```python
from build123d import *


with BuildPart() as f1:
    # F0 (on Right) → F1 (revolve)
    with BuildSketch(Plane.YZ):
        with BuildLine():
            Line((-6.35, -10.473485), (-5.488451, -10.473485))
            Line((-5.488451, -10.473485), (-5.488451, -3.844697))
            Line((-5.488451, -3.844697), (0, -3.844697))
            Line((0, -3.844697), (0, -1.438863))
            Line((0, -1.438863), (-10.85, -1.438863))
            ThreePointArc((-10.85, -1.438863), (-11.91066, -1.878203), (-12.35, -2.938863))
            Line((-12.35, -2.938863), (-12.35, -3.438863))
            Line((-12.35, -3.438863), (-6.35, -3.438863))
            Line((-6.35, -3.438863), (-6.35, -6.318287))
            Line((-6.35, -6.318287), (-6.35, -9.81605))
            Line((-6.35, -9.81605), (-6.35, -10.473485))
        make_face()
        Polygon((-6.45, -7.265888), (-6.35, -9.81605), (-6.35, -6.318287), align=None)
    revolve(axis=Axis((0, 0, 16.107956), (0, 0, 1)))


solid = f1.part
```
Model file for the job. Use its own axes, mm. A direction names the side the tool comes from. Give positions to 0.01 mm unless a question says otherwise; leave off trailing zeros. Loops run counter-clockwise (first coordinate to the right, second up) from the corner with the lowest first, then second, coordinate; pieces in that order, holes last. Notation, with made-up numbers: (-2, 15) -> (17, 15) arc R24 cw to (17, 46) -> close; hole circle Ø4 at (64, 86.25). An arc over 180 degrees is marked (long way). Use CSV: the item, a comma, the result in double quotes. Start each with the question number.
1) Slice it at C-C on z = -7.75. Give the cut face in (x, y).
2) Slice it at A-A on y = 0. Give the cut face in (x, z), plus the area to 3 significant figures.
3) Tool access for faces 1 (the cylindrical face through (3.71, -11.78, -3.19)), 2 (the cylindrical face through (-6.2, 1.38, -10.15)), 3 (the cylindrical face through (-6.2, 1.38, -4.9)): list every direction of +Z, -Z, +X, -X, +Y, -Y with a clear straight run to the whole face (end or side of a thin tool).
4) Mould opens along Y. For faces 4 (the flat face through (3, 6, -3.439)), 5 (the cylindrical face through (1.649, -5.235, -7.113)), 6 (the conical face through (-3.887, 5.069, -8.842)) say: released by +Y, released by -Y, zero draft, split by the parting line, or undercut.
5) Wall check: line 1 (Y direction, x = -1.5, z = -7.25); line 2 (Z direction, x = 2.25, y = 0.25); line 3 (X direction, y = 4.75, z = -7). Give the ranges that are in metal, low to high.
6) Flat gauge pins, fed straight in: pin 1 Ø3 at (y, z) = (-4, -2.5) entering from -X; pin 2 Ø3.5 at (x, y) = (1.5, 2.5) entering from -Z. Where does each tip first touch, or does it go through?
Computed values:
1,outline,"circle Ø12.86 at (0, 0); hole circle Ø10.98 at (0, 0)"
2,outline,"(-12.35, -3.44) -> (-6.35, -3.44) -> (-6.35, -6.32) -> (-6.45, -7.27) -> (-6.35, -9.82) -> (-6.35, -10.47) -> (-5.49, -10.47) -> (-5.49, -3.84) -> (5.49, -3.84) -> (5.49, -10.47) -> (6.35, -10.47) -> (6.35, -9.82) -> (6.45, -7.27) -> (6.35, -6.32) -> (6.35, -3.44) -> (12.35, -3.44) -> (12.35, -2.94) arc R1.5 ccw to (10.85, -1.44) -> (-10.85, -1.44) arc R1.5 ccw to (-12.35, -2.94) -> close"
2,area,"65.4 mm^2"
3,face 1,"+Z, -Z"
3,face 2,"-Z"
3,face 3,"none"
4,face 4,"zero draft"
4,face 5,"undercut"
4,face 6,"split by the parting line"
5,line 1,"y = -6.27 to -5.28, 5.28 to 6.27"
5,line 2,"z = -3.84 to -1.44"
5,line 3,"x = -4.32 to -2.75, 2.75 to 4.32"
6,pin 1,"stops at x = -12.08"
6,pin 2,"stops at z = -3.84"
